Design review of the part built by this model. Coordinates are the model's own, in mm. A direction names the side the tool comes from. Round coordinates to 2 decimals unless told otherwise and drop trailing zeros. Order: outer loops, then holes, each group sorted by start corner. A loop starts at its lowest first (then second) coordinate and runs counter-clockwise, first axis right, second up. Notation, with made-up numbers: (4.5, 49.5) - (17.5, 49.5) arc R16 ccw to (17.5, 60.5) - close; hole circle Ø9 at (-21.75, -3.5). An arc over 180 degrees is marked (long way). Write item = value, one per line.
from build123d import *

# Parameters (mm, degrees)
SKETCH_4_W          = 130
SKETCH_4_H          = 80
EXTRUDE_3_DEPTH     = 15
SKETCH_5_R          = 17.5
CUT_EXTRUDE_1_DEPTH = 2
SKETCH_6_R          = 13
CUT_EXTRUDE_2_DEPTH = 10
SKETCH_7_R          = 6
CUT_EXTRUDE_3_DEPTH = 78.420927403


with BuildPart() as part:
    # Эскиз4 → Бобышка-Вытянуть3 (new body)
    with BuildSketch(Plane(origin=(0, 0, 0), x_dir=(1, 0, 0), z_dir=(0, 1, 0))):
        Rectangle(SKETCH_4_W, SKETCH_4_H)
    extrude(amount=EXTRUDE_3_DEPTH)

    # Эскиз5 → Вырез-Вытянуть1 (cut)
    with BuildSketch(Plane(origin=(0, 15, 0), x_dir=(1, 0, 0), z_dir=(0, 1, 0))):
        with Locations(Location((0, 0, 0), (0, 0, 270))):
            Circle(SKETCH_5_R)
    extrude(amount=-CUT_EXTRUDE_1_DEPTH, mode=Mode.SUBTRACT)

    # Эскиз6 → Вырез-Вытянуть2 (cut)
    with BuildSketch(Plane.XZ):
        with Locations(Location((0, 0, 0), (0, 0, 270))):
            Circle(SKETCH_6_R)
    extrude(amount=-CUT_EXTRUDE_2_DEPTH, mode=Mode.SUBTRACT)

    # Эскиз7 → Вырез-Вытянуть3 (cut, through all)
    with BuildSketch(Plane(origin=(0, 13, 0), x_dir=(1, 0, 0), z_dir=(0, 1, 0))):
        with Locations(Location((0, 0, 0), (0, 0, 270))):
            Circle(SKETCH_7_R)
    extrude(amount=-CUT_EXTRUDE_3_DEPTH, mode=Mode.SUBTRACT)


solid = part.part
Item 1: Take a section at C-C, the plane y = 5.25. State the section outline as (x, z) points.
Data:
outline = (-65, -40) - (65, -40) - (65, 40) - (-65, 40) - close; hole circle Ø26 at (0, 0)
Item 2: Insertion check: P1, Ø3, axis at x = 20.5, z = 4.5, coming from the -Y side; P2, Ø21, axis at x = 0, z = 0, coming from the +Y side; P3, Ø11, axis at x = 0, z = 0, coming from the +Y side; P4, Ø15.5, axis at x = 0, z = 0, coming from the -Y side. Each pin has a flat end and moves straight along its axis. Give the tip position at first contact, or say it passes through.
Data:
P1 = 0
P2 = 13
P3 = through
P4 = 10
Item 3: Take a section at A-A, the plane z = 0. State the section outline as (x, y) points, and give its area (3 significant figures).
Data:
outline = (-65, 0) - (-13, 0) - (-13, 10) - (-6, 10) - (-6, 13) - (-17.5, 13) - (-17.5, 15) - (-65, 15) - close; (6, 10) - (13, 10) - (13, 0) - (65, 0) - (65, 15) - (17.5, 15) - (17.5, 13) - (6, 13) - close
area = 1,580 mm2
Item 4: For faces 1 (the face through (-15, 0, -1)), 2 (the face through (-8, 13, 0)), 3 (the face through (-3, 10, -6)), list the 3-axis set-ups (+Z, -Z, +X, -X, +Y, -Y) from which the entire face can be reached by the end or side of a thin tool; tool diameter is ignored.
Data:
face_1 = +Z, -Z, +X, -X, -Y
face_2 = +Y
face_3 = -Y
Item 5: For line 1 along X through (y, z) = (2.5, 0); line 2 along X through (y, z) = (13.9, 0); line 3 along Y through (x, z) = (11, -7), list the stretches that pass through material, from the lowest coordinate up. Write a range as [from, to].
Data:
line_1 = [-65, -13], [13, 65]
line_2 = [-65, -17.5], [17.5, 65]
line_3 = [0, 13]
Item 6: Take a section at B-B, the plane x = 0. State the section outline as (y, z) points.
Data:
outline = (0, -40) - (15, -40) - (15, -17.5) - (13, -17.5) - (13, -6) - (10, -6) - (10, -13) - (0, -13) - close; (0, 13) - (10, 13) - (10, 6) - (13, 6) - (13, 17.5) - (15, 17.5) - (15, 40) - (0, 40) - close
Item 7: The part is to be moulded in two halves that separate along Z. For faces 4 (the face through (65, 7, 1)), 5 (the face through (-7.91, 4.93, 10.316)), 6 (the face through (-1, 7, 40)), say which applies: +Z half, -Z half, draft (parallel to the pull), parting line (faces both ways), or undercut.
Data:
face_4 = draft
face_5 = undercut
face_6 = +Z half
